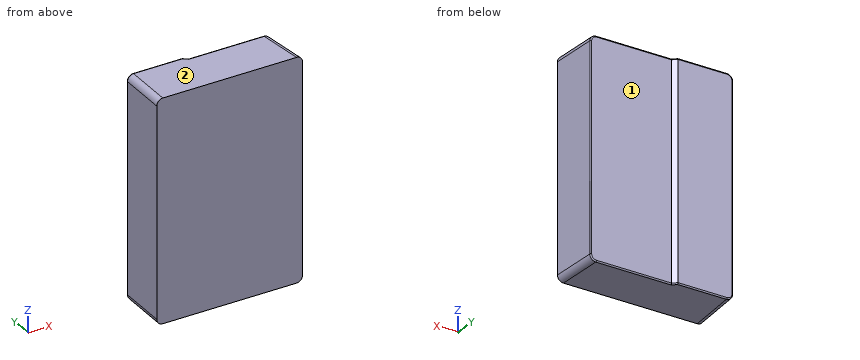
from build123d import *

# Parameters (mm, degrees)
PAD_DEPTH   = 90
FILLET_R    = 5
FILLET001_R = 1


with BuildPart() as part:
    # Sketch → Pad (new body, symmetric)
    with BuildSketch(Plane.XY):
        Polygon((51.85, 39.5), (119.35, 39.5), (121.7, 0), (0, 0), (2.35, 42.5), (48.35, 42.5), align=None)
    extrude(amount=PAD_DEPTH, both=True)

    # Fillet
    fillet_edges = [part.edges().sort_by_distance(p)[0] for p in [
        (120.525, 19.75, 90),
        (1.175, 21.25, 90),
        (120.525, 19.75, -90),
        (1.175, 21.25, -90),
    ]]
    fillet(fillet_edges, radius=FILLET_R)

    # Fillet001
    fillet001_edges = [part.edges().sort_by_distance(p)[0] for p in [
        (83.09558, 39.5, 90),
        (50.1, 41, 90),
        (27.853819, 42.5, 90),
        (3.818055, 42.5, 88.536883),
        (2.35, 42.5, 0),
        (3.818055, 42.5, -88.536883),
        (27.853819, 42.5, -90),
        (50.1, 41, -90),
        (83.09558, 39.5, -90),
        (117.88138, 39.5, -88.537095),
        (119.35, 39.5, 0),
        (117.88138, 39.5, 88.537095),
    ]]
    fillet(fillet001_edges, radius=FILLET001_R)


solid = part.part
Could you check a few things on this model? Use its own coordinates, in mm. Face numbers are marked on the shaded views. A direction names the side the tool comes from. Give positions to 0.01 mm unless a question says otherwise; leave off trailing zeros. Loops run counter-clockwise (first coordinate to the right, second up) from the corner with the lowest first, then second, coordinate; pieces in that order, holes last. Notation, with made-up numbers: (50, 23) -> (108, 23) arc R28 ccw to (108, 61) -> close; hole circle Ø2 at (87.25, 23). An arc over 180 degrees is marked (long way). Return JSON: item names as keys, results as strings.
Item 1: Which directions (+Z, -Z, +X, -X, +Y, -Y) give clear straight access to the entire face, cutting with the end or side of a thin tool? Please do the marked faces 1 and 2.
Geometry results:
{"face 1": "+Z, -Z, +X, +Y", "face 2": "+Z, +X, -X, +Y, -Y"}
Item 2: I'm going to push flat-ended pins straight in: pin 1 (5 mm diameter, centred on y = 12, z = 43, fed in from +X); pin 2 (20 mm diameter, centred on x = 84, z = 40.5, fed in from +Y); pin 3 (1.5 mm diameter, centred on y = 22.5, z = -33, fed in from +X). Where does each tip first touch, or does it pass through?
Geometry results:
{"pin 1": "stops at x = 121.13", "pin 2": "stops at y = 39.5", "pin 3": "stops at x = 120.41"}
Item 3: I need wall thicknesses on L1, parallel to Y at x = 109, z = -51.5; L2, parallel to X at y = 41, z = 60.5; L3, parallel to X at y = 36, z = 82. Which ranges of each line are inside material? Lowest first, please. Write a range as from..to.
Geometry results:
{"L1": "y = 0..39.5", "L2": "x = 2.27..50.1", "L3": "x = 1.99..119.56"}
Item 4: If we section it at A-A on x = 63: List the corners of the cut face in (y, z) for me, plus the area to 3 significant figures.
Geometry results:
{"outline": "(0, -90) -> (38.5, -90) arc R1 ccw to (39.5, -89) -> (39.5, 89) arc R1 ccw to (38.5, 90) -> (0, 90) -> close", "area": "7,110 mm²"}
Item 5: If we section it at B-B on z = -53.5: List the corners of the cut face in (x, y) for me.
Geometry results:
{"outline": "(0, 0) -> (121.7, 0) -> (119.41, 38.56) arc R1 ccw to (118.41, 39.5) -> (51.85, 39.5) -> (48.35, 42.5) -> (3.3, 42.5) arc R1 ccw to (2.3, 41.56) -> close"}
